from build123d import *

# Parameters (mm, degrees)
F0_W     = 12
F0_H     = 30
F1_DEPTH = 200
F2_R     = 1
F3_R     = 2.75
F4_DEPTH = 4
F5_DEPTH = 12.001


with BuildPart() as f1:
    # F0 (on Right) → F1 (new body, symmetric)
    with BuildSketch(Plane.YZ):
        with Locations((6, 15)):
            Rectangle(F0_W, F0_H)
    extrude(amount=F1_DEPTH, both=True)

    # F2
    f2_edges = [f1.edges().sort_by_distance(p)[0] for p in [
        (-200, 6, 30),
        (200, 6, 30),
        (200, 6, 0),
        (-200, 6, 0),
    ]]
    fillet(f2_edges, radius=F2_R)

    # F3 (on face) → F4 (cut)
    with BuildSketch(Plane.XZ):
        with BuildLine():
            Line((3.4641016151, 17), (3.0594010768, 17.7009618943))
            ThreePointArc((3.0594010768, 17.7009618943), (2.3094010768, 19), (0.8094010768, 19))
            Line((0.8094010768, 19), (0, 19))
            Line((0, 19), (-0.8094010768, 19))
            ThreePointArc((-0.8094010768, 19), (-2.3094010768, 19), (-3.0594010768, 17.7009618943))
            Line((-3.0594010768, 17.7009618943), (-3.4641016151, 17))
            Line((-3.4641016151, 17), (-3.8688021535, 16.2990381057))
            ThreePointArc((-3.8688021535, 16.2990381057), (-4.6188021535, 15), (-3.8688021535, 13.7009618943))
            Line((-3.8688021535, 13.7009618943), (-3.4641016151, 13))
            Line((-3.4641016151, 13), (-3.0594010768, 12.2990381057))
            ThreePointArc((-3.0594010768, 12.2990381057), (-2.3094010768, 11), (-0.8094010768, 11))
            Line((-0.8094010768, 11), (0, 11))
            Line((0, 11), (0.8094010768, 11))
            ThreePointArc((0.8094010768, 11), (2.3094010768, 11), (3.0594010768, 12.2990381057))
            Line((3.0594010768, 12.2990381057), (3.4641016151, 13))
            Line((3.4641016151, 13), (3.8688021535, 13.7009618943))
            ThreePointArc((3.8688021535, 13.7009618943), (4.6188021535, 15), (3.8688021535, 16.2990381057))
            Line((3.8688021535, 16.2990381057), (3.4641016151, 17))
        make_face()
        with Locations((0, 15)):
            Circle(F3_R, mode=Mode.SUBTRACT)
    extrude(amount=-F4_DEPTH, mode=Mode.SUBTRACT)

    # F5 (cut, through all): a face of the model
    f5_faces = [f1.faces().sort_by_distance(p)[0] for p in [
        (0, 0, 15),
    ]]
    extrude(f5_faces, amount=-F5_DEPTH, mode=Mode.SUBTRACT)


solid = f1.part
The listing builds one solid part. Answer for the finished solid, in the listing's coordinates (mm). Coordinates: 2 decimals unless noted, no trailing zeros.
Q1. Given P1, Ø5, axis at x = 0, z = 15, coming from the -Y side; P2, Ø10, axis at x = -158, z = 6.5, coming from the -Y side, each flat-ended and moving along its own axis, determine where each tip first touches the part or whether it passes through.
Q2. For a pull along Z with two mould halves and no side action, classify faces 1 (the face through (200, 6, 15)), 2 (the face through (3, 6, 0)), 3 (the face through (3, 6, 30)), 4 (the face through (0, 4, 18)) as pulls with the +Z half, pulls with the -Z half, needs draft (parallel to the pull), parting line crosses it, or undercut.
Q3. Consider line 1 (Z direction, x = 0, y = 8.25). Determine where the line is inside the solid, lowest interval first.
Answers follow:
1. P1: passes through
1. P2: stops at y = 0
2. face 1: needs draft
2. face 2: pulls with the -Z half
2. face 3: pulls with the +Z half
2. face 4: undercut
3. line 1: z = 0 to 12.25, 17.75 to 30
